Here's how the part is built. I have some questions about the finished solid (model axes, mm). A direction names the side the tool comes from. Give positions to 0.01 mm unless a question says otherwise; leave off trailing zeros. Loops run counter-clockwise (first coordinate to the right, second up) from the corner with the lowest first, then second, coordinate; pieces in that order, holes last.
Q1. Suppose I cut it at D-D (x = 2.5). List the corners of the cut face in (y, z) for me.
Q2. Suppose I cut it at A-A (z = -8.75). List the corners of the cut face in (x, y) for me, and give its area (3 significant figures).
Q3. Suppose I cut it at C-C (z = -3.5). List the corners of the cut face in (x, y) for me.
Q4. I need wall thicknesses on probe 1 along X at (y, z) = (1.1, -4); probe 2 along Z at (x, y) = (1, 0.6); probe 3 along X at (y, z) = (0.65, -12). Which ranges of each line are inside material? Lowest first, please.
Q5. For faces 1 (the face through (5.707, 0.626, -7.917)), 2 (the face through (0.18, 0.64, -0.05)), 3 (the face through (2.893, 0.626, -12.303)), which set-ups out of +Z, -Z, +X, -X, +Y, -Y let a thin tool reach every point of the face, with its end or its side?
Q6. Thinking about a two-plate mould opening in X: for faces 4 (the face through (0, 1, -7)), 5 (the face through (0.753, 0.626, -15.205)), 6 (the face through (0.254, 1, -7)), which applies, pulls with the +X half, pulls with the -X half, needs draft (parallel to the pull), parting line crosses it, or undercut?
Q7. I'm going to push a flat-ended pin straight in: P1, Ø0.6, axis at y = 1, z = -5.5, coming from the -X side. Where does the tip first touch, or does it pass through?
```python
from build123d import *

# Parameters (mm, degrees)
BOSS_EXTRUDE1_DEPTH = 1.27
FILLET1_R           = 1.27


with BuildPart() as part:
    # Sketch1 → Boss-Extrude1 (new body)
    with BuildSketch(Plane(origin=(0, 0, 0), x_dir=(1, 0, 0), z_dir=(0, 1, 0))):
        with BuildLine():
            Line((0, 0), (0, 14.224))
            ThreePointArc((0, 14.224), (0.77136744, 15.210108975), (1.914194705, 14.698870794))
            Line((1.914194705, 14.698870794), (4.288548676, 10.207897267))
            ThreePointArc((4.288548676, 10.207897267), (4.486671136, 9.850723748), (4.698989351, 9.501801969))
            Line((4.698989351, 9.501801969), (6.744540566, 6.287487077))
            ThreePointArc((6.744540566, 6.287487077), (6.815438139, 5.328506429), (6.055012218, 4.739929527))
            Line((6.055012218, 4.739929527), (6.013106646, 4.990448833))
            ThreePointArc((6.013106646, 4.990448833), (6.583426086, 5.43188151), (6.530252906, 6.151116996))
            Line((6.530252906, 6.151116996), (4.484701691, 9.365431888))
            ThreePointArc((4.484701691, 9.365431888), (4.267075521, 9.723076711), (4.064, 10.089179569))
            Line((4.064, 10.089179569), (1.689646029, 14.580153096))
            ThreePointArc((1.689646029, 14.580153096), (0.83252558, 14.963581731), (0.254, 14.224))
            Line((0.254, 14.224), (0.254, -0.200987113))
            ThreePointArc((0.254, -0.200987113), (0.204269521, -0.959727605), (0.352610056, -0.213969373))
            Line((0.352610056, -0.213969373), (0.418350094, 0.031375786))
            ThreePointArc((0.418350094, 0.031375786), (0.301490909, -1.215208728), (0, 0))
        make_face()
    extrude(amount=BOSS_EXTRUDE1_DEPTH)

    # Fillet1
    fillet1_edges = [part.edges().sort_by_distance(p)[0] for p in [
        (0.254, 0.635, 0.200987113),
        (0, 0.635, 0),
    ]]
    fillet(fillet1_edges, radius=FILLET1_R)


solid = part.part
```
Solutions:
1. outline: (0, -13.59) - (1.27, -13.59) - (1.27, -13.05) - (0, -13.05) - close
2. outline: (0, 0) - (0.25, 0) - (0.25, 1.27) - (0, 1.27) - close; (4.88, 0) - (5.18, 0) - (5.18, 1.27) - (4.88, 1.27) - close
2. area: 0.705 mm2
3. outline: (0, 0) - (0.25, 0) - (0.25, 1.27) - (0, 1.27) - close
4. probe 1: x = 0 to 0.25
4. probe 2: z = -15.24 to -14.99
4. probe 3: x = 0 to 0.25, 3.05 to 3.34
5. face 1: -Z, +X, +Y, -Y
5. face 2: +Y, -Y
5. face 3: +Z, +Y, -Y
6. face 4: pulls with the -X half
6. face 5: parting line crosses it
6. face 6: undercut
7. P1: stops at x = 0
